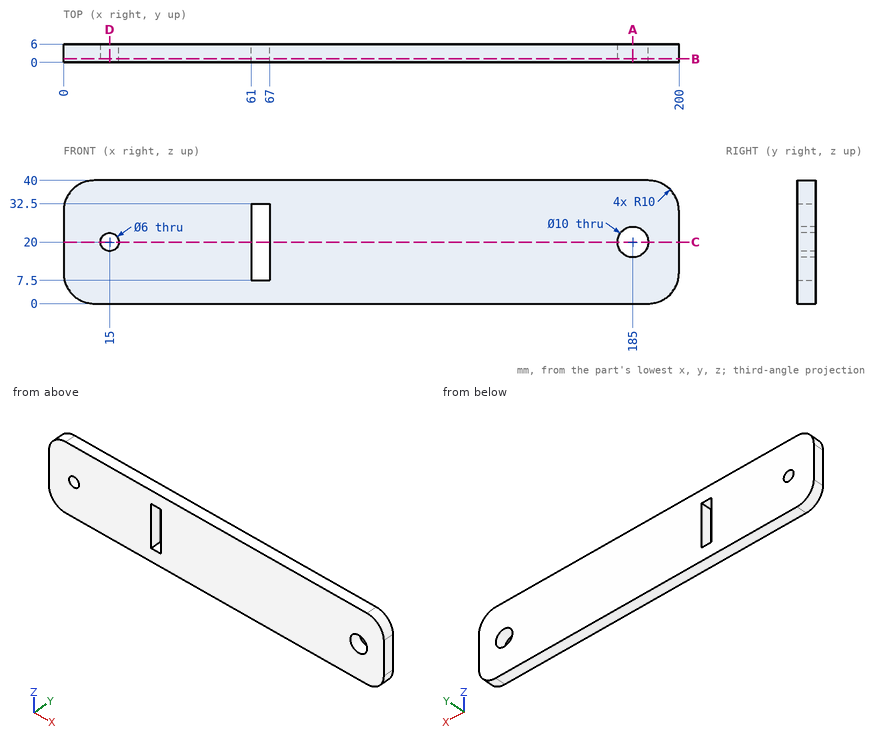
The figure shows three views and two pictorial views of one solid part (mm, origin at its lowest corner). Answer the questions. Give positions to 0.01 mm unless a question says otherwise; leave off trailing zeros. Write each loop counter-clockwise with the first axis right and the second up, starting at its lowest first coordinate (ties: lowest second). Pieces come first, ordered by that corner, then holes.
Q1. Given pin 1 (5 mm diameter, centred on x = 15, z = 20, fed in from -Y); pin 2 (2 mm diameter, centred on y = 2.5, z = 33.5, fed in from +X); pin 3 (1 mm diameter, centred on y = 4, z = 8, fed in from -X), each flat-ended and moving along its own axis, determine where each tip first touches the part or whether it passes through.
Answer:
pin 1: passes through
pin 2: stops at x = 199.68
pin 3: stops at x = 0.11
Q2. The part is cut by section B-B on y = 1.2. Give the vertices of the cut face in (x, z).
Answer:
outline: (0, 10) arc R10 ccw to (10, 0) - (190, 0) arc R10 ccw to (200, 10) - (200, 30) arc R10 ccw to (190, 40) - (10, 40) arc R10 ccw to (0, 30) - close; hole circle Ø6 at (15, 20); hole (61, 7.5) - (67, 7.5) - (67, 32.5) - (61, 32.5) - close; hole circle Ø10 at (185, 20)
Q3. The part is cut by section A-A on x = 185. Give the vertices of the cut face in (y, z), and give its area (3 significant figures).
Answer:
outline: (0, 0) - (6, 0) - (6, 15) - (0, 15) - close; (0, 25) - (6, 25) - (6, 40) - (0, 40) - close
area: 180 mm2
Q4. The part is cut by section C-C on z = 20. Give the vertices of the cut face in (x, y), and give its area (3 significant figures).
Answer:
outline: (0, 0) - (12, 0) - (12, 6) - (0, 6) - close; (18, 0) - (61, 0) - (61, 6) - (18, 6) - close; (67, 0) - (180, 0) - (180, 6) - (67, 6) - close; (190, 0) - (200, 0) - (200, 6) - (190, 6) - close
area: 1,070 mm2
Q5. Straight lines are drawn through the part: L1, parallel to X at y = 4.1, z = 20; L2, parallel to Z at x = 15, y = 2.6; L3, parallel to X at y = 3.3, z = 24. For each, find the intervals that lie inside material, in ascending order.
Answer:
L1: x = 0 to 12, 18 to 61, 67 to 180, 190 to 200
L2: z = 0 to 17, 23 to 40
L3: x = 0 to 61, 67 to 182, 188 to 200
Q6. The part is cut by section D-D on x = 15. Give the vertices of the cut face in (y, z), and give its area (3 significant figures).
Answer:
outline: (0, 0) - (6, 0) - (6, 17) - (0, 17) - close; (0, 23) - (6, 23) - (6, 40) - (0, 40) - close
area: 204 mm2
